Can you work these out from the model? Positions are in its coordinate system, mm. A direction names the side the tool comes from. Round coordinates to 2 decimals unless told otherwise and drop trailing zeros. Loops run counter-clockwise (first coordinate to the right, second up) from the corner with the lowest first, then second, coordinate; pieces in that order, holes last. Notation, with made-up numbers: M 16.25,58 L 44.25,58 A21 ccw 44.25,94 Z; hole C 42,51.5 d7. An arc over 180 degrees is marked long. Answer as CSV lines item,"result".
from build123d import *

# Parameters (mm, degrees)
F0_R     = 9.525
F1_DEPTH = 787.4
F4_START = 127
F0_W     = 584.2
F0_H     = 330.2
F4_DEPTH = 12.7
F5_START = 431.8
F5_DEPTH = 12.7
F6_START = 711.2
F6_DEPTH = 12.7


with BuildPart() as f1:
    # F0 (on Top) → F1 (new body)
    with BuildSketch(Plane.XY):
        with Locations((-266.7, 139.7)):
            Circle(F0_R)
    extrude(amount=F1_DEPTH)


with BuildPart() as f2_1:
    # F2: instance of F1
    add(f1.part.mirror(Plane.XZ))


with BuildPart() as f3_1:
    # F3: instance of F1
    add(f1.part.mirror(Plane.YZ))


with BuildPart() as f3_2:
    # F3: instance of F2_1
    add(f2_1.part.mirror(Plane.YZ))


with BuildPart() as f1_1:
    add(f1.part)

    add(f2_1.part)  # F4 merges F2_1

    add(f3_1.part)  # F4 merges F3_1

    add(f3_2.part)  # F4 merges F3_2
    # F0 (on Top) → F4 (join)
    with BuildSketch(Plane.XY.offset(F4_START)):
        Rectangle(F0_W, F0_H)
        with Locations((-266.7, 139.7)):
            Circle(F0_R, mode=Mode.SUBTRACT)
    extrude(amount=F4_DEPTH)

    # F0 (on Top) → F5 (join)
    with BuildSketch(Plane.XY.offset(F5_START)):
        Rectangle(F0_W, F0_H)
        with Locations((-266.7, 139.7)):
            Circle(F0_R, mode=Mode.SUBTRACT)
    extrude(amount=F5_DEPTH)

    # F0 (on Top) → F6 (join)
    with BuildSketch(Plane.XY.offset(F6_START)):
        Rectangle(F0_W, F0_H)
        with Locations((-266.7, 139.7)):
            Circle(F0_R, mode=Mode.SUBTRACT)
    extrude(amount=F6_DEPTH)


solid = f1_1.part
Item 1: If we section it at B-B on x = -129: Write out the boundary of the cut face in (y, z).
Output:
outline,"M -165.1,127 L 165.1,127 L 165.1,139.7 L -165.1,139.7 Z; M -165.1,431.8 L 165.1,431.8 L 165.1,444.5 L -165.1,444.5 Z; M -165.1,711.2 L 165.1,711.2 L 165.1,723.9 L -165.1,723.9 Z"
Item 2: If we section it at C-C on z = 670.5: Write out the boundary of the cut face in (x, y) (3 decimals).
Output:
outline,"C -266.7,-139.7 d19.05; C -266.7,139.7 d19.05; C 266.7,-139.7 d19.05; C 266.7,139.7 d19.05"
Item 3: If we section it at A-A on y = 43: Write out the boundary of the cut face in (x, z).
Output:
outline,"M -292.1,127 L 292.1,127 L 292.1,139.7 L -292.1,139.7 Z; M -292.1,431.8 L 292.1,431.8 L 292.1,444.5 L -292.1,444.5 Z; M -292.1,711.2 L 292.1,711.2 L 292.1,723.9 L -292.1,723.9 Z"
Item 4: If we section it at D-D on y = -139.7: State how many separate pieces and enclosed holes the cut face has, then the cut area to 3 significant figures.
Output:
separate pieces,"1"
enclosed holes,"2"
area,"50,800 mm2"
Item 5: Will this pin go through, and if not, where does the flat tip stop? pin 1 (1 mm diameter, centred on x = -175.5, y = 48.5, fed in from -Z).
Output:
pin 1,"stops at z = 127"
Item 6: If I drill on line 1 along Z through (x, y) = (3.5, 74.5); line 2 along X through (y, z) = (131, 229), over which ranges is the centre line in solid material (lowest first)? Write a range as from..to.
Output:
line 1,"z = 127..139.7, 431.8..444.5, 711.2..723.9"
line 2,"x = -270.58..-262.82, 262.82..270.58"
Item 7: We'd pull the mould along Y, two halves only. Please class faces 6 (the face through (-276.216, -140.119, 62.611)), 7 (the face through (267, 140, 0)): released by +Y, released by -Y, zero draft, split by the parting line, or undercut.
Output:
face 6,"undercut"
face 7,"zero draft"
Item 8: On a 3-axis mill with a long thin cutter (end or side, diameter ignored), from which of +Z, -Z, +X, -X, +Y, -Y can I reach the whole of each face in a straight line? I mean faces 1 (the face through (-276.216, -140.119, 283.705)), 2 (the face through (-267, 140, 787.4)), 3 (the face through (-276.216, -140.119, 755.206)), 4 (the face through (276.216, -140.119, 62.611)), 5 (the face through (-267, 140, 0)). Say none if no direction works.
Output:
face 1,"none"
face 2,"+Z, +X, -X, +Y, -Y"
face 3,"+Z"
face 4,"-Z"
face 5,"-Z, +X, -X, +Y, -Y"
